The drawing under review shows one solid part. Ordinate dimensions are in mm from its lowest x, y, z. Give positions to 0.01 mm unless a question says otherwise; leave off trailing zeros. Loops run counter-clockwise (first coordinate to the right, second up) from the corner with the lowest first, then second, coordinate; pieces in that order, holes last. Notation, with made-up numbers: (-20.5, 75) - (-4.5, 75) arc R13 cw to (-4.5, 89) - close; hole circle Ø10 at (53.5, -29.5). An arc over 180 degrees is marked (long way). Write each question's results on one line, items separated by ' | '.
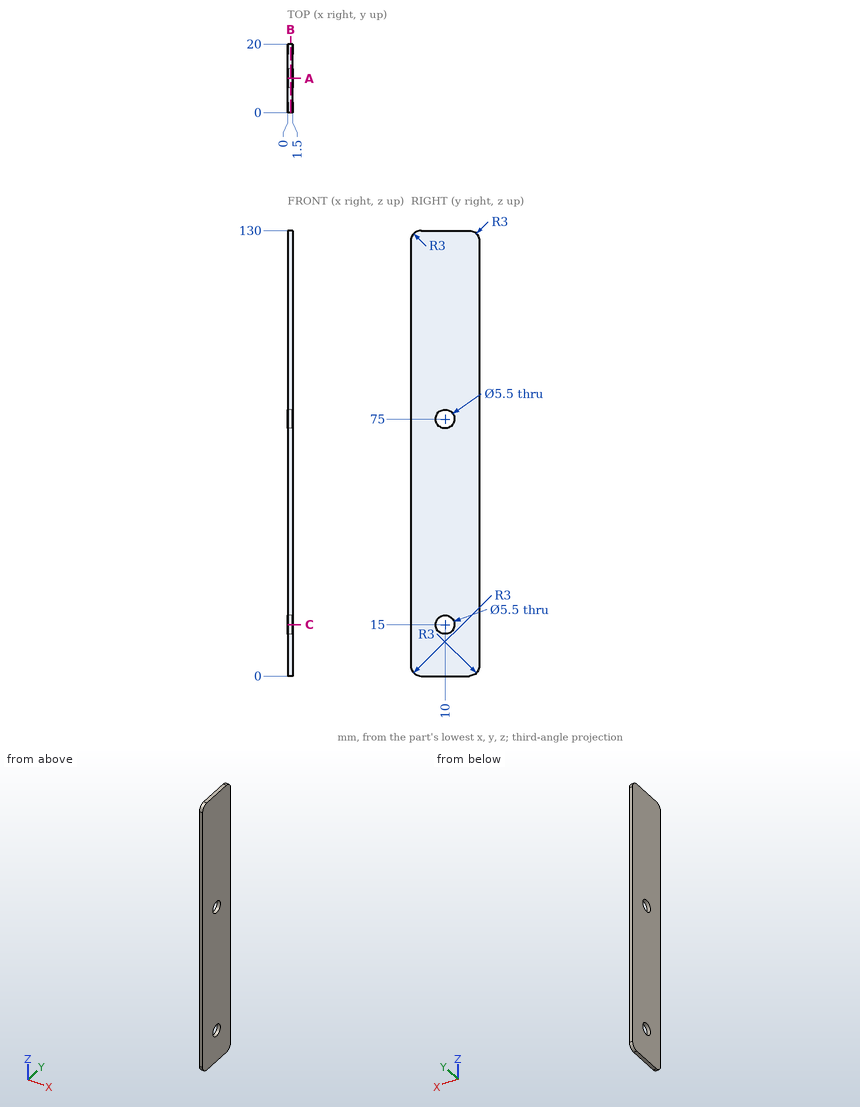
(1) Take a section at C-C on z = 15. Give the boundary of the cut face in (x, y).
Answers below:
outline: (0, 0) - (1.5, 0) - (1.5, 7.25) - (0, 7.25) - close; (0, 12.75) - (1.5, 12.75) - (1.5, 20) - (0, 20) - close
(2) Wall thickness on line 1 along Y through (x, z) = (1.15, 15); line 2 along Z through (x, y) = (0.4, 8.25); line 3 along Z through (x, y) = (1.25, 7.75): over which ranges is each line inside the solid? List them lowest first. Write a range as from..to.
Answers below:
line 1: 0..7.25, 12.75..20 | line 2: 0..12.88, 17.12..72.88, 77.12..130 | line 3: 0..13.42, 16.58..73.42, 76.58..130
(3) Take a section at A-A on y = 10. Give the boundary of the cut face in (x, z), plus the area to 4 significant figures.
Answers below:
outline: (0, 0) - (1.5, 0) - (1.5, 12.25) - (0, 12.25) - close; (0, 17.75) - (1.5, 17.75) - (1.5, 72.25) - (0, 72.25) - close; (0, 77.75) - (1.5, 77.75) - (1.5, 130) - (0, 130) - close | area: 178.5 mm2
(4) Take a section at B-B on x = 0.85. Give the boundary of the cut face in (y, z), plus the area to 3 significant figures.
Answers below:
outline: (0, 3) arc R3 ccw to (3, 0) - (17, 0) arc R3 ccw to (20, 3) - (20, 127) arc R3 ccw to (17, 130) - (3, 130) arc R3 ccw to (0, 127) - close; hole circle Ø5.5 at (10, 15); hole circle Ø5.5 at (10, 75) | area: 2,540 mm2
(5) Insertion check: P1, Ø5, axis at y = 10, z = 15, coming from the +X side. The pin has a flat end and moves straight along its axis. Give the tip position at first contact, or say it passes through.
Answers below:
P1: through
